Read the model definition and answer for the solid it produces. Units are mm, in the model's axes. A direction names the side the tool comes from. Coordinates: 2 decimals unless noted, no trailing zeros. Write each loop counter-clockwise with the first axis right and the second up, starting at its lowest first coordinate (ties: lowest second). Pieces come first, ordered by that corner, then holes. Notation, with made-up numbers: (24, 57) - (65, 57) arc R36 ccw to (65, 93) - close; hole circle Ø4 at (70.25, 62). An arc over 180 degrees is marked (long way). Return JSON: item names as keys, results as strings.
```python
from build123d import *

# Parameters (mm, degrees)
F0_R     = 5
F1_DEPTH = 3
F3_DEPTH = 20
F5_DEPTH = 2
F6_W     = 5
F6_H     = 5
F7_DEPTH = 5


with BuildPart() as f1:
    # F0 (on Front) → F1 (new body)
    with BuildSketch(Plane.XZ):
        with BuildLine():
            Line((7.5, -12.5), (7.5, 0))
            ThreePointArc((7.5, 0), (0, 7.5), (-7.5, 0))
            Line((-7.5, 0), (-7.5, -12.5))
            Line((-7.5, -12.5), (7.5, -12.5))
        make_face()
        Circle(F0_R, mode=Mode.SUBTRACT)
    extrude(amount=F1_DEPTH)

    # F2 (on Front) → F3 (join)
    with BuildSketch(Plane.XZ):
        with BuildLine():
            Line((10.5, -12.5), (10.5, 0))
            ThreePointArc((10.5, 0), (0, 10.5), (-10.5, 0))
            Line((-10.5, 0), (-10.5, -12.5))
            Line((-10.5, -12.5), (-7.5, -12.5))
            Line((-7.5, -12.5), (-7.5, 0))
            ThreePointArc((-7.5, 0), (0, 7.5), (7.5, 0))
            Line((7.5, 0), (7.5, -12.5))
            Line((7.5, -12.5), (10.5, -12.5))
        make_face()
    extrude(amount=F3_DEPTH)

    # F4 (on face) → F5 (join)
    with BuildSketch(Plane.XZ.offset(20)):
        with BuildLine():
            Line((10.5, -12.5), (10.5, 0))
            ThreePointArc((10.5, 0), (0, 10.5), (-10.5, 0))
            Line((-10.5, 0), (-10.5, -12.5))
            Line((-10.5, -12.5), (10.5, -12.5))
        make_face()
    extrude(amount=F5_DEPTH)

    # F6 (on face) → F7 (cut)
    with BuildSketch(Plane(origin=(-10.5, 0, 0), x_dir=(0, -1, 0), z_dir=(-1, 0, 0))):
        with Locations((17.5, -5)):
            Rectangle(F6_W, F6_H)
    extrude(amount=-F7_DEPTH, mode=Mode.SUBTRACT)


solid = f1.part
```
(1) A cutting plane is placed at D-D (y = -5). Determine the outline of the cut face in (x, z).
Answer:
{"outline": "(-10.5, -12.5) - (-7.5, -12.5) - (-7.5, 0) arc R7.5 cw to (7.5, 0) - (7.5, -12.5) - (10.5, -12.5) - (10.5, 0) arc R10.5 ccw to (-10.5, 0) - close"}
(2) Determine the mould class of faces 1 (the face through (0, -20, -2)), 2 (the face through (10.5, -11, -6)), 3 (the face through (0, -22, -1)) for opening direction Y: +Y half, -Y half, draft (parallel to the pull), parting line (faces both ways), or undercut.
Answer:
{"face 1": "undercut", "face 2": "draft", "face 3": "-Y half"}
(3) A cutting plane is placed at B-B (z = -9). Determine the outline of the cut face in (x, y), and give its area (3 significant figures).
Answer:
{"outline": "(-10.5, -22) - (10.5, -22) - (10.5, 0) - (-10.5, 0) - close; hole (-7.5, -20) - (7.5, -20) - (7.5, -3) - (-7.5, -3) - close", "area": "207 mm²"}
(4) A cutting plane is placed at A-A (x = 0). Determine the outline of the cut face in (y, z), and give its area (3 significant figures).
Answer:
{"outline": "(-22, -12.5) - (-20, -12.5) - (-20, 7.5) - (-3, 7.5) - (-3, 5) - (0, 5) - (0, 10.5) - (-22, 10.5) - close; (-3, -12.5) - (0, -12.5) - (0, -5) - (-3, -5) - close", "area": "136 mm²"}
(5) Straight lines are drawn through the part: line 1 (Y direction, x = -3.75, z = -11.25); line 2 (Z direction, x = 0, y = -1.6); line 3 (X direction, y = -9.5, z = -9). For each, find the intervals that lie inside material, in ascending order. Write a range as from..to.
Answer:
{"line 1": "-22..-20, -3..0", "line 2": "-12.5..-5, 5..10.5", "line 3": "-10.5..-7.5, 7.5..10.5"}
(6) Flat-ended cylindrical pins translate along their axes: P1, Ø0.9, axis at x = -9, y = -18.5, coming from the +Z side; P2, Ø1, axis at x = -6, y = -9, coming from the -Z side; P3, Ø4, axis at x = -5.5, y = -15.5, coming from the +Z side. Find the tip coordinate at first contact, or state that the pin passes through.
Answer:
{"P1": "z = 6.09", "P2": "z = 3.74", "P3": "z = 9.9"}
(7) A cutting plane is placed at C-C (y = -16). Determine the outline of the cut face in (x, z), and give its area (3 significant figures).
Answer:
{"outline": "(-10.5, -12.5) - (-7.5, -12.5) - (-7.5, -7.5) - (-10.5, -7.5) - close; (-10.5, -2.5) - (-7.5, -2.5) - (-7.5, 0) arc R7.5 cw to (7.5, 0) - (7.5, -12.5) - (10.5, -12.5) - (10.5, 0) arc R10.5 ccw to (-10.5, 0) - close", "area": "145 mm²"}
(8) Which of the six approach directions +Z, -Z, +X, -X, +Y, -Y give full straight-line access (tool end or side, diameter ignored) to faces 4 (the face through (9, -11, -12.5)), 5 (the face through (-10.5, -11, -6)), 6 (the face through (-1.08, -1.48, -4.88)), 7 (the face through (0, -3, -7)), 8 (the face through (-9, -17, -2.5))?
Answer:
{"face 4": "-Z, +X, -X, +Y, -Y", "face 5": "+Z, -Z, -X, +Y, -Y", "face 6": "+Y", "face 7": "-Z", "face 8": "-X"}
